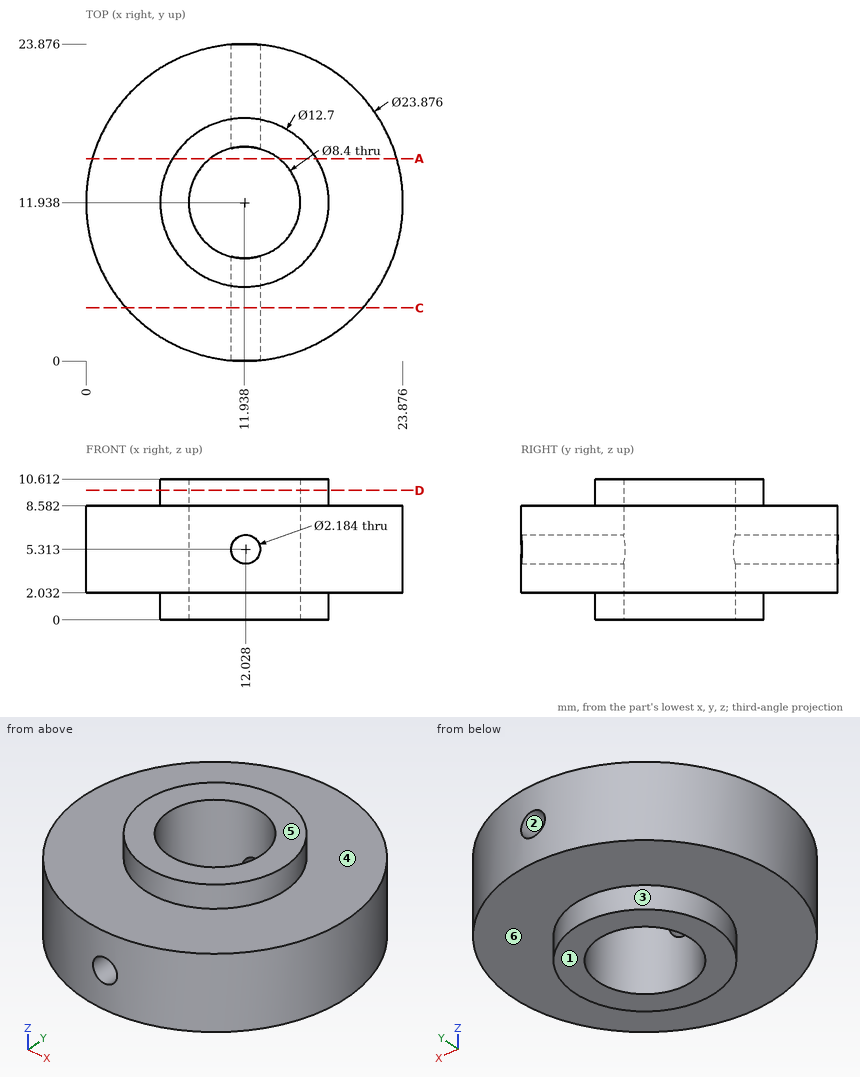
Input: dimensioned drawing with shaded views. Units: mm. Origin: part minimum x, y, z. A direction names the side the tool comes from. Give positions to 0.01 mm unless a question says otherwise; leave off trailing zeros. Write each loop counter-clockwise with the first axis right and the second up, starting at its lowest first coordinate (ties: lowest second). Pieces come first, ordered by that corner, then holes. Notation, with made-up numbers: (65.25, -19) - (102.25, -19) arc R5 cw to (102.25, -10) - close; hole circle Ø7 at (-31.75, -33). An arc over 180 degrees is marked (long way). Write item = value, one per line. Start each with the question number.
1) Pin query (flat end, axial travel): pin 1 (3 mm diameter, centred on x = 4, z = 9, fed in from +Y). Return the tip coordinate at first contact, or that it passes through.
2) Reachability of the marked faces 4, 5 and 6 from +Z, -Z, +X, -X, +Y, -Y: full face, straight path, thin tool, end or side. Return the list, or none.
3) Draft query along X for the marked faces 1, 2 and 3. Return one class per face: pulls with the +X half, pulls with the -X half, needs draft (parallel to the pull), parting line crosses it, or undercut.
4) Cut plane C-C (y = 4). Return loops of the section in (x, z) (1 decimal), and give its area (3 significant figures).
5) Cut plane D-D (z = 9.75). Return loops of the section in (x, y).
6) Material intervals for L1, parallel to Z at x = 12, y = 7.25 (1 decimal); L2, parallel to X at y = 13, z = 5.5 (1 decimal); L3, parallel to X at y = 14, z = 5 (1 decimal), sorted ascending. Write a range as [from, to].
7) Cut plane A-A (y = 15.25). Return loops of the section in (x, z) (1 decimal).
Answers follow:
q1.pin_1 = 21.95
q2.face_4 = +Z
q2.face_5 = +Z, +X, -X, +Y, -Y
q2.face_6 = -Z
q3.face_1 = needs draft
q3.face_2 = undercut
q3.face_3 = parting line crosses it
q4.outline = (3, 2) - (20.9, 2) - (20.9, 8.6) - (3, 8.6) - close; hole circle Ø2.2 at (12, 5.3)
q4.area = 113 mm^2
q5.outline = circle Ø12.7 at (11.94, 11.94); hole circle Ø8.4 at (11.94, 11.94)
q6.L1 = [0, 4.2], [6.4, 10.6]
q6.L2 = [0, 7.9], [16, 23.8]
q6.L3 = [0.2, 8.3], [15.6, 23.7]
q7.outline = (0.5, 2) - (6.5, 2) - (6.5, 0) - (9.4, 0) - (9.4, 10.6) - (6.5, 10.6) - (6.5, 8.6) - (0.5, 8.6) - close; (14.5, 0) - (17.4, 0) - (17.4, 2) - (23.4, 2) - (23.4, 8.6) - (17.4, 8.6) - (17.4, 10.6) - (14.5, 10.6) - close
